```python
from build123d import *

# Parameters (mm, degrees)
F0_R     = 30
F1_DEPTH = 8
F2_T     = -2.5
F3_R     = 22.5
F4_DEPTH = 25
F5_R     = 2
F6_R     = 2


with BuildPart() as f1:
    # F0 (on Front) → F1 (new body)
    with BuildSketch(Plane.XZ):
        Circle(F0_R)
    extrude(amount=F1_DEPTH)

    # F2
    f2_openings = [f1.faces().sort_by_distance(p)[0] for p in [
        (0, -8, 0),
    ]]
    offset(amount=F2_T, openings=f2_openings)

    # F3 (on face) → F4 (cut)
    with BuildSketch(Plane(origin=(0, 0, 0), x_dir=(-1, 0, 0), z_dir=(0, 1, 0))):
        Circle(F3_R)
    extrude(amount=-F4_DEPTH, mode=Mode.SUBTRACT)

    # F5
    f5_edges = [f1.edges().sort_by_distance(p)[0] for p in [
        (-30, 0, 0),
    ]]
    fillet(f5_edges, radius=F5_R)

    # F6
    f6_edges = [f1.edges().sort_by_distance(p)[0] for p in [
        (-27.5, -2.5, 0),
    ]]
    fillet(f6_edges, radius=F6_R)


solid = f1.part
```
Part model, mm, in its own coordinate system. A direction names the side the tool comes from. Round coordinates to 2 decimals unless told otherwise and drop trailing zeros. Loops run counter-clockwise (first coordinate to the right, second up) from the corner with the lowest first, then second, coordinate; pieces in that order, holes last. Notation, with made-up numbers: (47, 58.5) -> (67, 58.5) arc R15 cw to (67, 87.5) -> close; hole circle Ø7 at (5, 13). An arc over 180 degrees is marked (long way). Use CSV: the item, a comma, the result in double quotes. Start each with the question number.
1) Cut at C-C, the plane y = -6.75. Write the cut outline in (x, z), plus the area to 3 significant figures.
2) Wall check: L1, parallel to Z at x = 0, y = -6.8; L2, parallel to X at y = -7, z = -23; L3, parallel to Z at x = 21, y = -4.75. Give the ranges that are in metal, low to high. Write a range as [from, to].
3) Which spindle directions (+Z, -Z, +X, -X, +Y, -Y) get a long thin tool onto all of the face, cutting with end or side? Do faces 1 (the flat face through (13.2, -8, -24.3)), 2 (the cylindrical face through (-5.961, -6.226, -26.846)). Say none if no direction does.
4) Drop flat-ended pins along their axis: P1, Ø4, axis at y = -5.5, z = -17.5, coming from the +X side; P2, Ø4, axis at x = 1, z = 23.5, coming from the -Y side; P3, Ø3, axis at x = -22, y = -4, coming from the -Z side. Give the stop position or say it passes through.
5) Cut at B-B, the plane x = 0. Write the cut outline in (y, z).
6) Cut at A-A, the plane z = 0. Write the cut outline in (x, y), plus the area to 3 significant figures.
Determined:
1,outline,"circle Ø60 at (0, 0); hole circle Ø55 at (0, 0)"
1,area,"452 mm2"
2,L1,"z = [-30, -27.5], [27.5, 30]"
2,L2,"x = [-19.26, -15.07], [15.07, 19.26]"
2,L3,"z = [-21.42, -17.76], [17.76, 21.42]"
3,face 1,"+Z, -Z, +X, -X, -Y"
3,face 2,"-Y"
4,P1,"stops at x = 25.69"
4,P2,"stops at y = -2.5"
4,P3,"stops at z = -21.9"
5,outline,"(-8, -30) -> (-2, -30) arc R2 ccw to (0, -28) -> (0, -22.5) -> (-2.5, -22.5) -> (-2.5, -25.5) arc R2 cw to (-4.5, -27.5) -> (-8, -27.5) -> close; (-8, 27.5) -> (-4.5, 27.5) arc R2 cw to (-2.5, 25.5) -> (-2.5, 22.5) -> (0, 22.5) -> (0, 28) arc R2 ccw to (-2, 30) -> (-8, 30) -> close"
6,outline,"(-30, -8) -> (-27.5, -8) -> (-27.5, -4.5) arc R2 cw to (-25.5, -2.5) -> (-22.5, -2.5) -> (-22.5, 0) -> (-28, 0) arc R2 ccw to (-30, -2) -> close; (22.5, -2.5) -> (25.5, -2.5) arc R2 cw to (27.5, -4.5) -> (27.5, -8) -> (30, -8) -> (30, -2) arc R2 ccw to (28, 0) -> (22.5, 0) -> close"
6,area,"65.0 mm2"
